Print and shaded views of the part. All mm, measured from the part's lowest x, y and z. A direction names the side the tool comes from. Round coordinates to 2 decimals unless told otherwise and drop trailing zeros. Order: outer loops, then holes, each group sorted by start corner. A loop starts at its lowest first (then second) coordinate and runs counter-clockwise, first axis right, second up. Notation, with made-up numbers: (61.5, -20.75) -> (92.5, -20.75) arc R32 cw to (92.5, 7.25) -> close; hole circle Ø5 at (0, 24). An arc over 180 degrees is marked (long way). Answer as CSV lines item,"result".
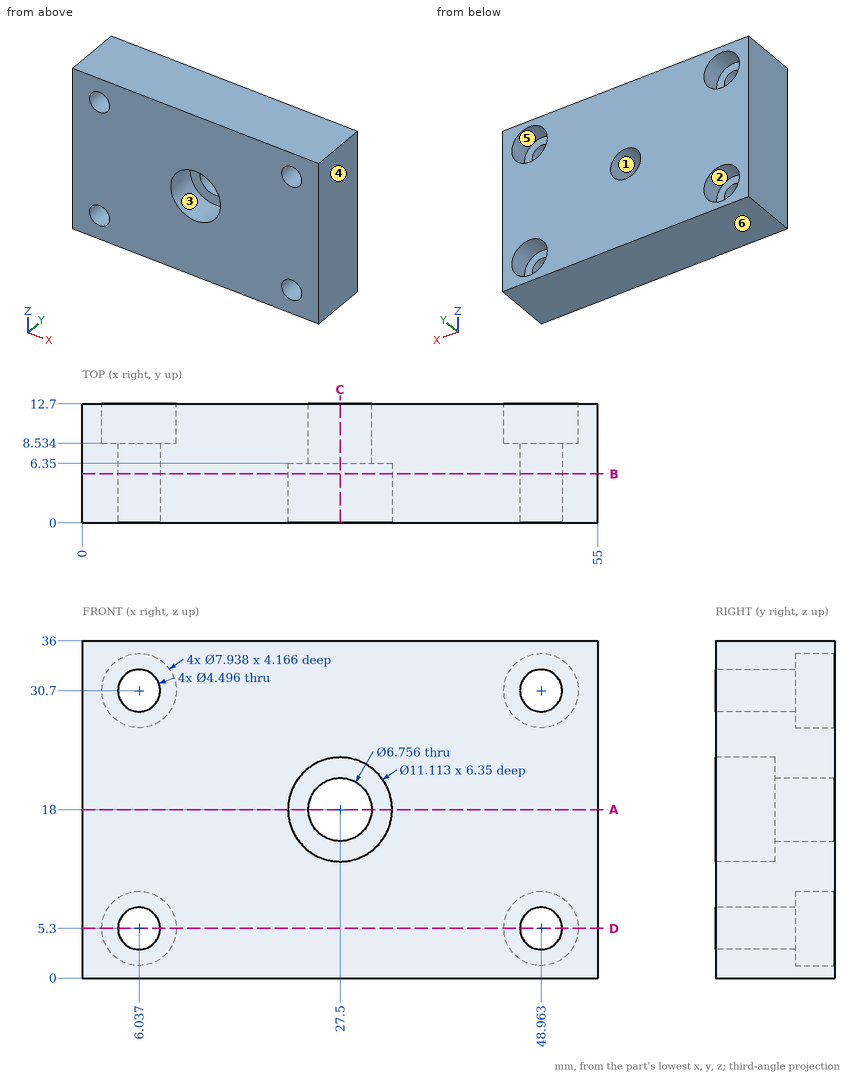
Q1. Tool access for the marked faces 1, 2 and 3: list every direction of +Z, -Z, +X, -X, +Y, -Y with a clear straight run to the whole face (end or side of a thin tool).
Checks:
face 1,"+Y, -Y"
face 2,"+Y"
face 3,"-Y"
Q2. Saw through at A-A (z = 18). Write the cut outline in (x, y), plus the area to 3 significant figures.
Checks:
outline,"(0, 0) -> (21.94, 0) -> (21.94, 6.35) -> (24.12, 6.35) -> (24.12, 12.7) -> (0, 12.7) -> close; (30.88, 6.35) -> (33.06, 6.35) -> (33.06, 0) -> (55, 0) -> (55, 12.7) -> (30.88, 12.7) -> close"
area,"585 mm²"
Q3. Flat gauge pins, fed straight in: pin 1 (2.5 mm diameter, centred on x = 47.5, z = 6, fed in from +Y); pin 2 (12.5 mm diameter, centred on x = 6.037, z = 5.3, fed in from +Y); pin 3 (4 mm diameter, centred on x = 27.5, z = 18, fed in from +Y); pin 4 (3.5 mm diameter, centred on x = 29, z = 16.5, fed in from -Y). Where does each tip first touch, or does it go through?
Checks:
pin 1,"y = 8.53"
pin 2,"y = 12.7"
pin 3,"through"
pin 4,"y = 6.35"
Q4. Mould opens along X. For the marked faces 4, 5 and 6 say: +X half, -X half, draft (parallel to the pull), parting line (faces both ways), or undercut.
Checks:
face 4,"+X half"
face 5,"undercut"
face 6,"draft"
Q5. Saw through at C-C (x = 27.5). Write the cut outline in (y, z).
Checks:
outline,"(0, 0) -> (12.7, 0) -> (12.7, 14.62) -> (6.35, 14.62) -> (6.35, 12.44) -> (0, 12.44) -> close; (0, 23.56) -> (6.35, 23.56) -> (6.35, 21.38) -> (12.7, 21.38) -> (12.7, 36) -> (0, 36) -> close"
Q6. Saw through at B-B (y = 5.25). Write the cut outline in (x, z) (1 decimal).
Checks:
outline,"(0, 0) -> (55, 0) -> (55, 36) -> (0, 36) -> close; hole circle Ø4.5 at (6, 5.3); hole circle Ø4.5 at (6, 30.7); hole circle Ø11.1 at (27.5, 18); hole circle Ø4.5 at (49, 5.3); hole circle Ø4.5 at (49, 30.7)"
Q7. Wall check: L1, parallel to Z at x = 49, y = 9.25; L2, parallel to Z at x = 52.5, y = 10 (1 decimal); L3, parallel to Z at x = 23, y = 4.25. Give the ranges that are in metal, low to high. Write a range as [from, to].
Checks:
L1,"[0, 1.33], [9.27, 26.73], [34.67, 36]"
L2,"[0, 3.5], [7.1, 28.9], [32.5, 36]"
L3,"[0, 14.74], [21.26, 36]"
Q8. Saw through at D-D (z = 5.3). Write the cut outline in (x, y) (1 decimal).
Checks:
outline,"(0, 0) -> (3.8, 0) -> (3.8, 8.5) -> (2.1, 8.5) -> (2.1, 12.7) -> (0, 12.7) -> close; (8.3, 0) -> (46.7, 0) -> (46.7, 8.5) -> (45, 8.5) -> (45, 12.7) -> (10, 12.7) -> (10, 8.5) -> (8.3, 8.5) -> close; (51.2, 0) -> (55, 0) -> (55, 12.7) -> (52.9, 12.7) -> (52.9, 8.5) -> (51.2, 8.5) -> close"
